Part model, mm, in its own coordinate system. Give positions to 0.01 mm unless a question says otherwise; leave off trailing zeros. Order: outer loops, then holes, each group sorted by start corner. A loop starts at its lowest first (then second) coordinate and runs counter-clockwise, first axis right, second up. Notation, with made-up numbers: M 35,37 L 44,37 A33 cw 44,65 Z; hole C 24,28 d3. An arc over 180 degrees is marked long. Answer as a JSON object with one key per item and string values.
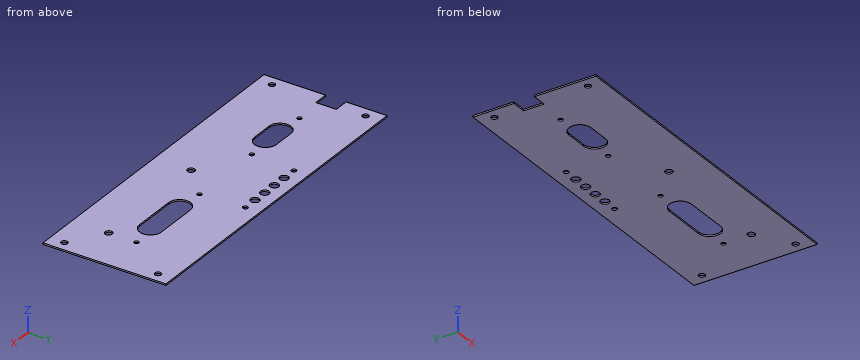
from build123d import *

# Parameters (mm, degrees)
SKETCH_1_W          = 228
SKETCH_1_H          = 84
SKETCH_1_R          = 2.15
EXTRUDE_1_DEPTH     = 1
SKETCH_4_R          = 1.6
SKETCH_4_W          = 14.464145402
SKETCH_4_H          = 14
CUT_EXTRUDE_2_DEPTH = 1
SKETCH_5_R          = 1.7
SKETCH_5_R_2        = 3
SKETCH_5_R_3        = 2.5
CUT_EXTRUDE_3_DEPTH = 10


with BuildPart() as part:
    # Эскиз1 → Вытянуть1 (new body)
    with BuildSketch(Plane.XY):
        Rectangle(SKETCH_1_W, SKETCH_1_H)
        with Locations((107, 32)):
            Circle(SKETCH_1_R, mode=Mode.SUBTRACT)
        with Locations(Location((-107, 32, 0), (0, 0, 180))):
            Circle(SKETCH_1_R, mode=Mode.SUBTRACT)
        with Locations((-107, -32)):
            Circle(SKETCH_1_R, mode=Mode.SUBTRACT)
        with Locations(Location((107, -32, 0), (0, 0, 180))):
            Circle(SKETCH_1_R, mode=Mode.SUBTRACT)
    extrude(amount=EXTRUDE_1_DEPTH)

    # Эскиз4 → Вырез-Вытянуть2 (cut)
    with BuildSketch(Plane.XY.offset(1)):
        with Locations((19, 2)):
            Circle(SKETCH_4_R)
        with Locations((84, 2)):
            Circle(SKETCH_4_R)
        with Locations((-84, 2)):
            Circle(SKETCH_4_R)
        with Locations((-35, 2)):
            Circle(SKETCH_4_R)
        with BuildLine():
            Line((36.5, 7.5), (66.5, 7.5))
            ThreePointArc((66.5, 7.5), (74, 0), (66.5, -7.5))
            Line((66.5, -7.5), (36.5, -7.5))
            ThreePointArc((36.5, -7.5), (29, 0), (36.5, 7.5))
        make_face()
        with BuildLine():
            Line((-67, 7.5), (-52, 7.5))
            ThreePointArc((-52, 7.5), (-44.5, 0), (-52, -7.5))
            Line((-52, -7.5), (-67, -7.5))
            ThreePointArc((-67, -7.5), (-74.5, 0), (-67, 7.5))
        make_face()
        with Locations((-111.232072701, 7)):
            Rectangle(SKETCH_4_W, SKETCH_4_H)
    extrude(amount=-CUT_EXTRUDE_2_DEPTH, mode=Mode.SUBTRACT)

    # Эскиз5 → Вырез-Вытянуть3 (cut)
    with BuildSketch(Plane.XY.offset(1)):
        with Locations((-33, 32)):
            Circle(SKETCH_5_R)
        with Locations((17, 32)):
            Circle(SKETCH_5_R)
        with Locations((7, 32)):
            Circle(SKETCH_5_R_2)
        with Locations((-3, 32)):
            Circle(SKETCH_5_R_2)
        with Locations((-13, 32)):
            Circle(SKETCH_5_R_2)
        with Locations((-23, 32)):
            Circle(SKETCH_5_R_2)
        with Locations((-1, -17)):
            Circle(SKETCH_5_R_3)
        with Locations((84, -17)):
            Circle(SKETCH_5_R_3)
    extrude(amount=-CUT_EXTRUDE_3_DEPTH, mode=Mode.SUBTRACT)


solid = part.part
1. Cut at C-C on z = 0.2. State how many separate pieces and enclosed holes the cut face has, plus the area to 3 significant figures.
Worked answers:
{"separate pieces": "1", "enclosed holes": "18", "area": "17,700 mm^2"}
2. Probe line 1 along Y through (x, z) = (107, 0.45); line 2 along Y through (x, z) = (-66, 0.15); line 3 along Y through (x, z) = (-1, 0.5). List the from-to ranges inside material, lowest first.
Worked answers:
{"line 1": "y = -42 to -34.15, -29.85 to 29.85, 34.15 to 42", "line 2": "y = -42 to -7.5, 7.5 to 42", "line 3": "y = -42 to -19.5, -14.5 to 29.76, 34.24 to 42"}
3. Cut at A-A on y = -17. Give the cut face in (x, z), plus the area to 3 significant figures.
Worked answers:
{"outline": "M -114,0 L -3.5,0 L -3.5,1 L -114,1 Z; M 1.5,0 L 81.5,0 L 81.5,1 L 1.5,1 Z; M 86.5,0 L 114,0 L 114,1 L 86.5,1 Z", "area": "218 mm^2"}
4. Cut at B-B on x = 7. Give the cut face in (y, z), plus the area to 3 significant figures.
Worked answers:
{"outline": "M -42,0 L 29,0 L 29,1 L -42,1 Z; M 35,0 L 42,0 L 42,1 L 35,1 Z", "area": "78.0 mm^2"}
5. Cut at D-D on x = -107. Give the cut face in (y, z).
Worked answers:
{"outline": "M -42,0 L -34.15,0 L -34.15,1 L -42,1 Z; M -29.85,0 L 0,0 L 0,1 L -29.85,1 Z; M 14,0 L 29.85,0 L 29.85,1 L 14,1 Z; M 34.15,0 L 42,0 L 42,1 L 34.15,1 Z"}
